For this review, take the finished solid that the model builds, in its own axes (mm). A direction names the side the tool comes from. Coordinates: 2 decimals unless noted, no trailing zeros. Write each loop counter-clockwise with the first axis right and the second up, starting at its lowest first coordinate (ties: lowest second). Pieces come first, ordered by that corner, then holes. Notation, with made-up numbers: M 45.25,88.25 L 99.25,88.25 A31 ccw 99.25,118.25 Z; hole C 67,88 d8. An arc over 180 degrees is marked long. One line per question, with ' | ' between items.
from build123d import *

# Parameters (mm, degrees)
BOSS_EXTRUDE1_DEPTH = 10
SKETCH2_W           = 30
SKETCH2_H           = 10
BOSS_EXTRUDE2_DEPTH = 60
SKETCH3_W           = 30
SKETCH3_H           = 10
BOSS_EXTRUDE3_DEPTH = 40


with BuildPart() as part:
    # Sketch1 → Boss-Extrude1 (new body)
    with BuildSketch(Plane.XY):
        Polygon((0, 0), (257.754406597, 0), (257.754406597, -27.219263415), (18.493720775, -27.219263415), (-56.767393161, -27.219263415), (-80, -27.219263415), (-85, -27.219263415), (-85, 0), (-80, 0), (-70, 0), align=None)
    extrude(amount=BOSS_EXTRUDE1_DEPTH)

    # Sketch2 → Boss-Extrude2 (add)
    with BuildSketch(Plane(origin=(0, -27.219263415, 0), x_dir=(-1, 0, 0), z_dir=(0, -1, 0))):
        with Locations((-242.754406597, -5)):
            Rectangle(SKETCH2_W, SKETCH2_H)
    extrude(amount=BOSS_EXTRUDE2_DEPTH)

    # Sketch3 → Boss-Extrude3 (add)
    with BuildSketch(Plane(origin=(0, -27.219263415, 0), x_dir=(-1, 0, 0), z_dir=(0, -1, 0))):
        with Locations((-112.754406597, -5)):
            Rectangle(SKETCH3_W, SKETCH3_H)
    extrude(amount=BOSS_EXTRUDE3_DEPTH)


solid = part.part
1. Machinability: for faces 1 (the flat face through (177, -27.219, 5)), 2 (the flat face through (5, -27.219, 5)), 3 (the flat face through (-85, -14, 5)), which of the approach directions +Z, -Z, +X, -X, +Y, -Y give a long, thin tool a straight path to every point of the face, cutting with its end or side? Answer none if there is none.
Computed values:
face 1: +Z, -Z, -Y | face 2: +Z, -Z, -X, -Y | face 3: +Z, -Z, -X, +Y, -Y
2. For line 1 along X through (y, z) = (-32.5, 0.5); line 2 along Y through (x, z) = (-42.5, 5.5); line 3 along X through (y, z) = (-80.5, 4), list the stretches that pass through material, from the lowest coordinate up.
Computed values:
line 1: x = 97.75 to 127.75, 227.75 to 257.75 | line 2: y = -27.22 to 0 | line 3: x = 227.75 to 257.75
3. Clearance check with flat-ended pins moving along their axes: P1, Ø3, axis at x = -5.5, z = 7, coming from the -Y side; P2, Ø5, axis at y = -34.5, z = 7, coming from the -X side; P3, Ø1, axis at y = -74, z = 8, coming from the -X side. State where each tip first meets the part, or that it passes through.
Computed values:
P1: stops at y = -27.22 | P2: stops at x = 97.75 | P3: stops at x = 227.75
4. Take a section at B-B on z = 8.5. State the section outline as (x, y) points.
Computed values:
outline: M -85,-27.22 L 97.75,-27.22 L 97.75,-67.22 L 127.75,-67.22 L 127.75,-27.22 L 227.75,-27.22 L 227.75,-87.22 L 257.75,-87.22 L 257.75,0 L -85,0 Z
5. Take a section at D-D on y = -79. State the section outline as (x, z) points.
Computed values:
outline: M 227.75,0 L 257.75,0 L 257.75,10 L 227.75,10 Z
6. Take a section at A-A on y = -46.5. State the section outline as (x, z) points.
Computed values:
outline: M 97.75,0 L 127.75,0 L 127.75,10 L 97.75,10 Z; M 227.75,0 L 257.75,0 L 257.75,10 L 227.75,10 Z
7. Take a section at C-C on x = 85. State the section outline as (y, z) points.
Computed values:
outline: M -27.22,0 L 0,0 L 0,10 L -27.22,10 Z
8. Draft analysis for pull direction X (two halves, no side actions). For faces 4 (the flat face through (127, -24, 0)), 5 (the flat face through (97.754, -47, 5)), 6 (the flat face through (227.754, -57, 5)), 7 (the flat face through (127.754, -47, 5)), state which applies: pulls with the +X half, pulls with the -X half, needs draft (parallel to the pull), parting line crosses it, or undercut.
Computed values:
face 4: needs draft | face 5: pulls with the -X half | face 6: undercut | face 7: undercut
